from build123d import *

# Parameters (mm, degrees)
F0_W     = 48.052
F0_H     = 48.052
F2_W     = 70
F2_H     = 70
F4_W     = 36.052
F4_H     = 36.052
F5_DEPTH = 38.1
F6_R     = 5
F7_W     = 48.052
F7_H     = 48.052
F8_DEPTH = 6


with BuildPart() as f3:
    # F0 (on Top) → F3 section 0
    with BuildSketch(Plane.XY):
        Rectangle(F0_W, F0_H)
    # F2 (on offset) → F3 section 1
    with BuildSketch(Plane.XY.offset(-127)):
        Rectangle(F2_W, F2_H)
    loft()

    # F4 (on face) → F5 (cut)
    with BuildSketch(Plane.XY):
        Rectangle(F4_W, F4_H)
    extrude(amount=-F5_DEPTH, mode=Mode.SUBTRACT)

    # F6
    f6_edges = [f3.edges().sort_by_distance(p)[0] for p in [
        (-29.513, -29.513, -63.5),
        (29.513, -29.513, -63.5),
        (-29.513, 29.513, -63.5),
        (29.513, 29.513, -63.5),
    ]]
    fillet(f6_edges, radius=F6_R)

    # F7 (on face) → F8 (cut)
    with BuildSketch(Plane(origin=(0, 0, -127), x_dir=(1, 0, 0), z_dir=(0, 0, -1))):
        Rectangle(F7_W, F7_H)
    extrude(amount=-F8_DEPTH, mode=Mode.SUBTRACT)


solid = f3.part
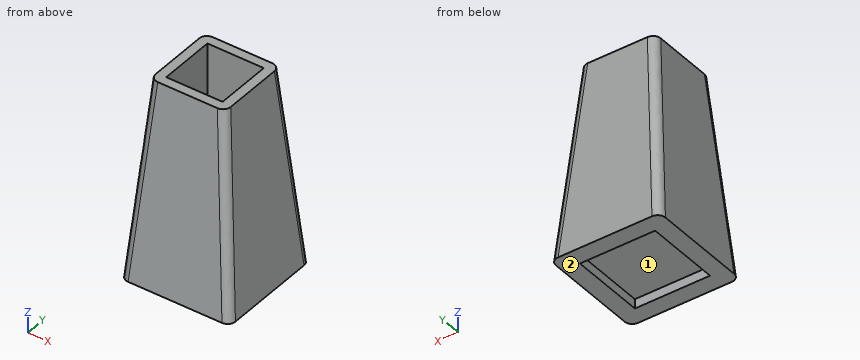
Design review of the part built by this model. Coordinates are the model's own, in mm. Face numbers are marked on the shaded views. Coordinates: 2 decimals unless noted, no trailing zeros. One line per item, written item: value.
1) To check wall thickness, follow probe 1 along Z at (x, y) = (-14, -15); probe 2 along Z at (x, y) = (20, -12); probe 3 along Y at (x, z) = (-13, -32). State the ranges of each line that lie inside material, in increasing order.
Answer sheet:
probe 1: z = -121 to -38.1
probe 2: z = -121 to 0
probe 3: y = -26.79 to -18.03, 18.03 to 26.79
2) Insertion check: pin 1 (5 mm diameter, centred on x = 11, z = -123.5, fed in from -Y); pin 2 (1.5 mm diameter, centred on y = -6, z = -104, fed in from -X); pin 3 (6.5 mm diameter, centred on x = 6, z = -123.5, fed in from +Y). Each pin has a flat end and moves straight along its axis. Give the tip position at first contact, or say it passes through.
Answer sheet:
pin 1: stops at y = -34.91
pin 2: stops at x = -33.08
pin 3: stops at y = 34.98
3) Mouldability with a two-part tool opening along Y and no side actions: class the marked faces 1 and 2 as +Y half, -Y half, draft (parallel to the pull), parting line (faces both ways), or undercut.
Answer sheet:
face 1: undercut
face 2: draft
